```python
from build123d import *

# Parameters (mm, degrees)
F0_R     = 10
F1_DEPTH = 30


with BuildPart() as f1:
    # F0 (on Front) → F1 (new body)
    with BuildSketch(Plane.XZ):
        with BuildLine():
            ThreePointArc((-32.5, -10), (-31.035534, -13.535534), (-27.5, -15))
            Line((-27.5, -15), (37.5, -15))
            Line((37.5, -15), (37.5, 0))
            Line((37.5, 0), (47.15451, 11.480002))
            Line((47.15451, 11.480002), (36.117656, 20.761832))
            Line((36.117656, 20.761832), (26.463146, 9.28183))
            Line((26.463146, 9.28183), (18.809811, 15.71817))
            Line((18.809811, 15.71817), (28.464321, 27.198172))
            Line((28.464321, 27.198172), (17.427467, 36.480002))
            Line((17.427467, 36.480002), (7.772957, 25))
            Line((7.772957, 25), (-2.227043, 25))
            Line((-2.227043, 25), (-2.227043, 15))
            Line((-2.227043, 15), (-7.227043, 15))
            Line((-7.227043, 15), (-7.227043, 25))
            Line((-7.227043, 25), (-22.227043, 25))
            ThreePointArc((-22.227043, 25), (-25.762577, 23.535534), (-27.227043, 20))
            Line((-27.227043, 20), (-27.227043, 5))
            Line((-27.227043, 5), (-27.5, 5))
            ThreePointArc((-27.5, 5), (-31.035534, 3.535534), (-32.5, 0))
            Line((-32.5, 0), (-32.5, -10))
        make_face()
        Circle(F0_R, mode=Mode.SUBTRACT)
    extrude(amount=F1_DEPTH)


solid = f1.part
```
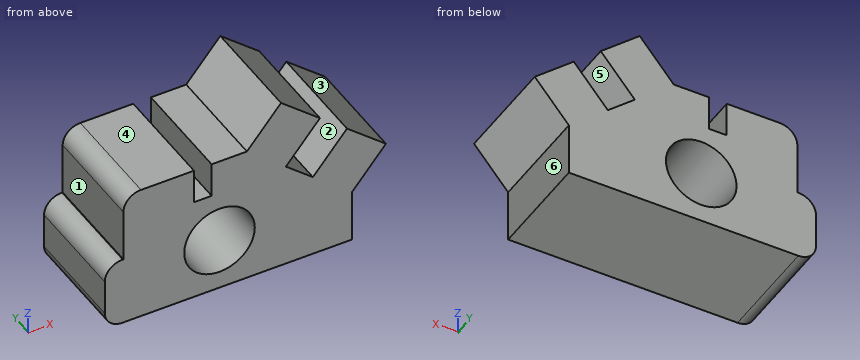
Source: CAD feature listing. Evaluate the final solid. Frame: model axes, mm. Face numbers are marked on the shaded views. A direction names the side the tool comes from. Give positions to 0.01 mm unless a question says otherwise; leave off trailing zeros. Loops run counter-clockwise (first coordinate to the right, second up) from the corner with the lowest first, then second, coordinate; pieces in that order, holes last. Notation, with made-up numbers: (31, 62.5) -> (60, 62.5) arc R21 ccw to (60, 84.5) -> close; hole circle Ø3 at (14.5, 87). An arc over 180 degrees is marked (long way). Put each result on its own line as item: value. Start each with the question number.
1) Cut plane C-C (z = -4.5). Return loops of the section in (x, y).
2) Cut plane D-D (x = -19.5). Return loops of the section in (y, z), then the cut area to 3 significant figures.
3) Cut plane B-B (y = -4.25). Return loops of the section in (x, z).
4) Contact query for flat-ended pins moving along their axis: P1, Ø5, axis at x = 3.5, y = -12, coming from the +Z side; P2, Ø2, axis at x = 30.5, y = -16.5, coming from the +Z side; P3, Ø7.5, axis at y = -18, z = 13.5, coming from the -X side. Output: stop coordinate, or through.
5) Cut plane A-A (x = 0). Return loops of the section in (y, z).
6) Reachability of the marked faces 4, 5 and 6 from +Z, -Z, +X, -X, +Y, -Y: full face, straight path, thin tool, end or side. Return the list, or none.
7) Draft query along Z for the marked faces 1, 2 and 3. Return one class per face: released by +Z, released by -Z, zero draft, split by the parting line, or undercut.
8) Material intervals for probe 1 along Z at (x, y) = (0, -15); probe 2 along X at (y, z) = (-14.75, 17); probe 3 along Z at (x, y) = (-15.5, -27.5), sorted ascending.
Results are:
1. outline: (-32.5, -30) -> (-8.93, -30) -> (-8.93, 0) -> (-32.5, 0) -> close; (8.93, -30) -> (37.5, -30) -> (37.5, 0) -> (8.93, 0) -> close
2. outline: (-30, -15) -> (0, -15) -> (0, 25) -> (-30, 25) -> close
2. area: 1,200 mm2
3. outline: (-32.5, -10) arc R5 ccw to (-27.5, -15) -> (37.5, -15) -> (37.5, 0) -> (47.15, 11.48) -> (36.12, 20.76) -> (26.46, 9.28) -> (18.81, 15.72) -> (28.46, 27.2) -> (17.43, 36.48) -> (7.77, 25) -> (-2.23, 25) -> (-2.23, 15) -> (-7.23, 15) -> (-7.23, 25) -> (-22.23, 25) arc R5 ccw to (-27.23, 20) -> (-27.23, 5) -> (-27.5, 5) arc R5 ccw to (-32.5, 0) -> close; hole circle Ø20 at (0, 0)
4. P1: stops at z = 25
4. P2: stops at z = 15.27
4. P3: stops at x = -27.23
5. outline: (-30, -15) -> (0, -15) -> (0, -10) -> (-30, -10) -> close; (-30, 10) -> (0, 10) -> (0, 25) -> (-30, 25) -> close
6. face 4: +Z, -X, +Y, -Y
6. face 5: +Y, -Y
6. face 6: -Z, +X, +Y, -Y
7. face 1: zero draft
7. face 2: undercut
7. face 3: released by +Z
8. probe 1: z = -15 to -10, 10 to 25
8. probe 2: x = -27.23 to -7.23, -2.23 to 19.89, 32.95 to 40.59
8. probe 3: z = -15 to 25
